Input: part model. Units: mm. Frame: model coordinates. Face numbers are marked on the shaded views. Round coordinates to 2 decimals unless told otherwise and drop trailing zeros. Loops run counter-clockwise (first coordinate to the right, second up) from the corner with the lowest first, then second, coordinate; pieces in that order, holes last. Notation, with made-up numbers: M -18.75,67 L 10.25,67 A9 cw 10.25,83 Z; hole C 59.25,14.5 d6. An arc over 180 degrees is marked long. Use one line per item in the form item = value. Start each with the question number.
Q1. Section query D-D, the plane x = 27.5. Output: boundary loops of the cut face in (y, z), and give its area (3 significant figures).
Q2. Section query C-C, the plane y = -27. Output: boundary loops of the cut face in (x, z).
Q3. Section query B-B, the plane z = 42.5. Output: boundary loops of the cut face in (x, y), and give its area (3 significant figures).
Q4. First-contact query: P1, Ø8, axis at x = -6, z = 86, coming from the +Y side; P2, Ø5, axis at x = -5, z = 19.5, coming from the +Y side; P3, Ø12, axis at x = 3, y = 15.5, coming from the -Z side. Flat tips, straight axial feed; report the tip coordinate or a pass-through.
Q5. Ray query, line 1 along Y through (x, z) = (-39, 75.5); line 2 along Y through (x, z) = (-32, 90); line 3 along Z through (x, y) = (-19.5, -9). Return the intervals inside material, ascending.
Q6. Section query A-A, the plane x = -16. Output: boundary loops of the cut face in (y, z).
Q7. Mould query, pull axis X, two halves, no side actions, for the marked faces 1, 2 and 3. Classes: pulls with the +X half, pulls with the -X half, needs draft (parallel to the pull), parting line crosses it, or undercut.
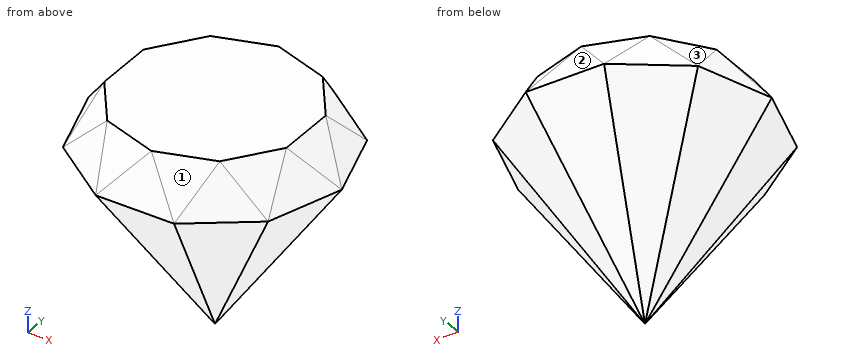
```python
from build123d import *

# Parameters (mm, degrees)
F5_DEPTH        = 20
F5_TAPER        = 29
F8_COPIES_COUNT = 10


# Not quite as in the source:
# - a pattern or mirror of a feature is missing from the dataset's text; its kind, count and spacing are read off the source's solid


with BuildPart() as f3:
    # F1 (on offset) → F3 section 0
    with BuildSketch(Plane.XY.offset(80), mode=Mode.PRIVATE) as f3_s0:
        Polygon((45.8155948031, -33.2869780703), (56.6311896062, 0), (45.8155948031, 33.2869780703), (17.5, 53.8594619006), (-17.5, 53.8594619006), (-45.8155948031, 33.2869780703), (-56.6311896062, 0), (-45.8155948031, -33.2869780703), (-17.5, -53.8594619006), (17.5, -53.8594619006), align=None)
    loft([Vertex(0, 0, 0), f3_s0.sketch])

    # F4 (on face) → F5 (join)
    with BuildSketch(Plane.XY.offset(80)):
        Polygon((45.8155948031, -33.2869780703), (56.6311896062, 0), (45.8155948031, 33.2869780703), (17.5, 53.8594619006), (-17.5, 53.8594619006), (-45.8155948031, 33.2869780703), (-56.6311896062, 0), (-45.8155948031, -33.2869780703), (-17.5, -53.8594619006), (17.5, -53.8594619006), align=None)
    extrude(amount=F5_DEPTH, taper=F5_TAPER)

    # F6 (on face) → F8 section 0
    with BuildSketch(Plane.XY.offset(100), mode=Mode.PRIVATE) as f8_s0:
        Polygon((44.9744890431, 0), (40.6798074962, 13.2176706945), (40.6798074962, -13.2176706945), align=None)
    f8 = loft([f8_s0.sketch, Vertex(56.6311896062, 0, 80)], mode=Mode.SUBTRACT)

    # F8_copies: F8 ×10 about axis
    f8_copies_axis = Axis((0, 0, 0), (0, 0, 1))
    for i in range(1, F8_COPIES_COUNT):
        add(f8.rotate(f8_copies_axis, i * 360 / F8_COPIES_COUNT), mode=Mode.SUBTRACT)


solid = f3.part
```
Results found:
q1.outline = M -46.59,80 L -19.98,48.02 L 0,38.85 L 19.98,48.02 L 46.59,80 L 34.45,97.72 L 31.36,100 L -31.36,100 L -34.45,97.72 Z
q1.area = 3,900 mm²
q2.outline = M -47.86,80 L -37.16,64.89 L -8.77,40.1 L 8.77,40.1 L 37.16,64.89 L 47.86,80 L 44.21,86.27 L 30.67,100 L -30.67,100 L -44.21,86.27 Z
q3.outline = M -30.09,0 L -24.34,-17.68 L -9.3,-28.61 L 9.3,-28.61 L 24.34,-17.68 L 30.09,0 L 24.34,17.68 L 9.3,28.61 L -9.3,28.61 L -24.34,17.68 Z
q3.area = 2,660 mm²
q4.P1 = 52.75
q4.P2 = 14.81
q4.P3 = 14.11
q5.line_1 = -34.49 to 34.49
q5.line_2 = -36.47 to 36.47
q5.line_3 = 31.68 to 100
q6.outline = M -53.86,80 L -49.24,73.14 L -11.62,27.94 L 0,22.6 L 11.62,27.94 L 49.24,73.14 L 53.86,80 L 52.91,81.71 L 37.57,100 L -37.57,100 L -52.91,81.71 Z
q7.face_1 = pulls with the +X half
q7.face_2 = needs draft
q7.face_3 = pulls with the -X half
